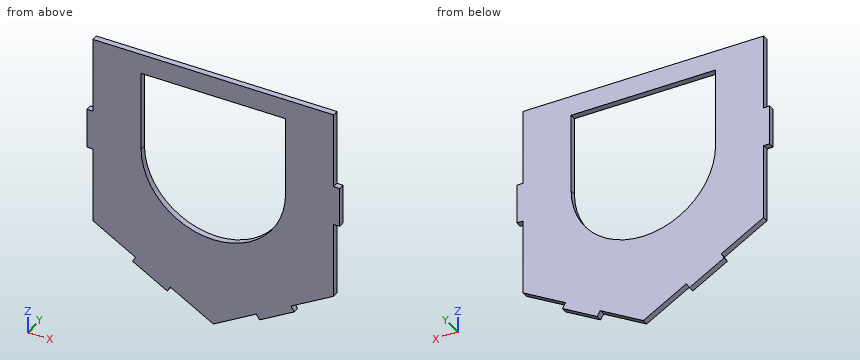
```python
from build123d import *

# Parameters (mm, degrees)
BOSS_EXTRUDE1_DEPTH = 15
CUT_EXTRUDE2_REACH  = 17


with BuildPart() as part:
    # Sketch1 → Boss-Extrude1 (new body)
    with BuildSketch(Plane(origin=(0, 0, 0), x_dir=(1, 0, 0), z_dir=(0, 1, 0))):
        Polygon((-300, -240), (300, -240), (300, -50), (315, -50), (315, 50), (300, 50), (300, 240), (193.911888036, 301.25), (201.411888036, 314.240381057), (114.809347658, 364.240381057), (107.309347658, 351.25), (0, 413.205080757), (-107.309347658, 351.25), (-114.809347658, 364.240381057), (-201.411888036, 314.240381057), (-193.911888036, 301.25), (-300, 240), (-300, 50), (-315, 50), (-315, -50), (-300, -50), align=None)
    extrude(amount=BOSS_EXTRUDE1_DEPTH)

    # Sketch2 → Cut-Extrude2 (cut, up to next)
    with BuildSketch(Plane(origin=(0, 15, 0), x_dir=(1, 0, 0), z_dir=(0, 1, 0)), mode=Mode.PRIVATE) as cut_extrude2_sk1:
        with BuildLine():
            Line((-180, -190), (180, -190))
            Line((180, -190), (180, 10))
            ThreePointArc((180, 10), (0, 190), (-180, 10))
            Line((-180, 10), (-180, -190))
        make_face()
    cut_extrude2_tool1 = extrude(cut_extrude2_sk1.sketch, amount=-CUT_EXTRUDE2_REACH, mode=Mode.PRIVATE) & part.part
    add(cut_extrude2_tool1.solids().sort_by_distance((0, 15, 16.950098))[0], mode=Mode.SUBTRACT)


solid = part.part
```
Check sheet for the modelled part. Datum: model origin and axes. Units: mm. Round coordinates to 2 decimals unless told otherwise and drop trailing zeros. Order: outer loops, then holes, each group sorted by start corner. A loop starts at its lowest first (then second) coordinate and runs counter-clockwise, first axis right, second up. Notation, with made-up numbers: (34.25, -25) -> (50.25, -25) arc R29 ccw to (50.25, 14) -> close; hole circle Ø2 at (-3, 8.25). An arc over 180 degrees is marked (long way). Use CSV: the item, a comma, the result in double quotes.
(1) Cross-section at D-D (x = 248). Record the boundary of the cut face in (y, z), and give its area (3 significant figures).
Worked out:
outline,"(0, -270.02) -> (15, -270.02) -> (15, 240) -> (0, 240) -> close"
area,"7,650 mm²"
(2) Cross-section at A-A (y = 3.25). Record the boundary of the cut face in (x, z), and give its area (3 significant figures).
Worked out:
outline,"(-315, -50) -> (-300, -50) -> (-300, -240) -> (-193.91, -301.25) -> (-201.41, -314.24) -> (-114.81, -364.24) -> (-107.31, -351.25) -> (0, -413.21) -> (107.31, -351.25) -> (114.81, -364.24) -> (201.41, -314.24) -> (193.91, -301.25) -> (300, -240) -> (300, -50) -> (315, -50) -> (315, 50) -> (300, 50) -> (300, 240) -> (-300, 240) -> (-300, 50) -> (-315, 50) -> close; hole (-180, -10) arc R180 ccw to (180, -10) -> (180, 190) -> (-180, 190) -> close"
area,"223,000 mm²"
(3) Material ranges on line 1 along X through (y, z) = (1.75, 55); line 2 along X through (y, z) = (4.5, -17); line 3 along X through (y, z) = (4, -354.5), recorded low to high. Write a range as from..to.
Worked out:
line 1,"-300..-180, 180..300"
line 2,"-315..-179.86, 179.86..315"
line 3,"-131.68..-109.19, -101.68..101.68, 109.19..131.68"
(4) Depth check by flat-ended pin: pin 1 (4.5 mm diameter, centred on x = -304, y = 10.5, fed in from -Z); pin 2 (4 mm diameter, centred on y = 6, z = -230.5, fed in from +X); pin 3 (4.5 mm diameter, centred on x = -32, y = 10, fed in from -Z). Enter the tip coordinate at first touch or a pass-through.
Worked out:
pin 1,"z = -50"
pin 2,"x = 300"
pin 3,"z = -396.03"
(5) Cross-section at B-B (z = 182). Record the boundary of the cut face in (x, y), and give its area (3 significant figures).
Worked out:
outline,"(-300, 0) -> (-180, 0) -> (-180, 15) -> (-300, 15) -> close; (180, 0) -> (300, 0) -> (300, 15) -> (180, 15) -> close"
area,"3,600 mm²"
(6) Cross-section at C-C (x = 42.5). Record the boundary of the cut face in (y, z).
Worked out:
outline,"(0, -388.67) -> (15, -388.67) -> (15, -184.91) -> (0, -184.91) -> close; (0, 190) -> (15, 190) -> (15, 240) -> (0, 240) -> close"
